Geometry check sheet. Reference: drawing and pictorial views, mm from the part's lowest x, y, z. Coordinates: 2 decimals unless noted, no trailing zeros. Loops run counter-clockwise (first coordinate to the right, second up) from the corner with the lowest first, then second, coordinate; pieces in that order, holes last. Notation, with made-up numbers: (16, 65) -> (44, 65) arc R28 ccw to (44, 102) -> close; hole circle Ø1 at (48, 38). An arc over 180 degrees is marked (long way). Use one line per item in the form item = value.
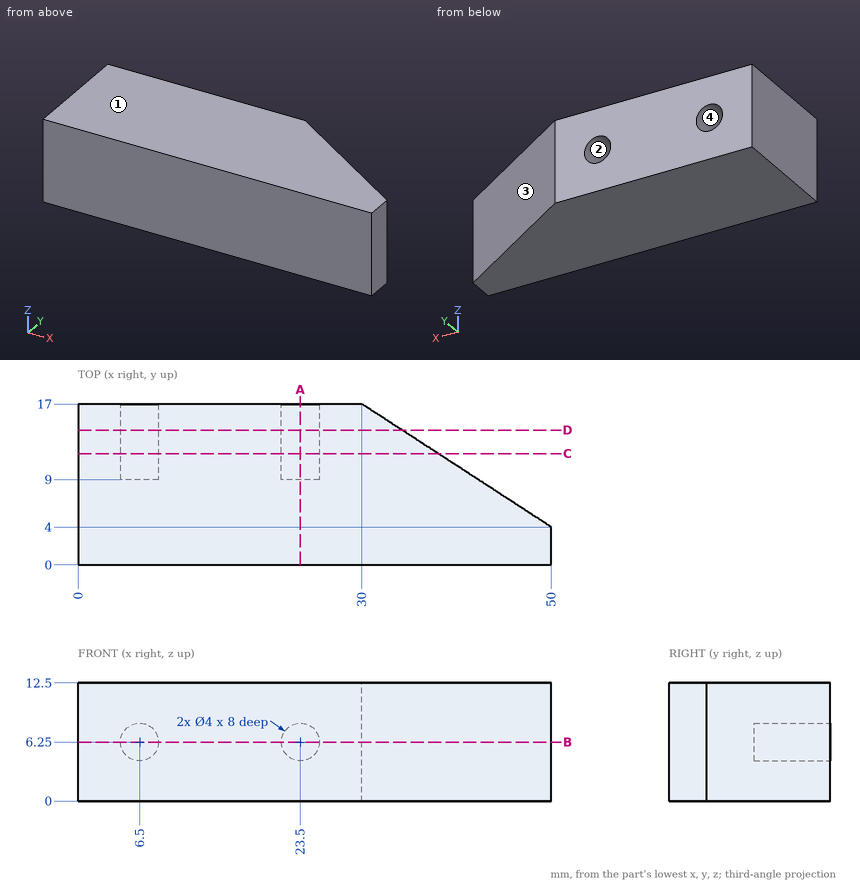
(1) Go/stop test with flat-tipped pins: P1, Ø4, axis at x = 42.5, z = 8.5, coming from the +Y side (3 decimals); P2, Ø5, axis at x = 39, z = 9, coming from the +Y side (3 decimals); P3, Ø3.5, axis at x = 23.5, z = 6.25, coming from the +Y side. Record where each tip stops, or that it passes through.
Established:
P1 = 10.175
P2 = 12.775
P3 = 9
(2) Section check A-A, the plane x = 23.5. Record the boundary of the cut face in (y, z).
Established:
outline = (0, 0) -> (17, 0) -> (17, 4.25) -> (9, 4.25) -> (9, 8.25) -> (17, 8.25) -> (17, 12.5) -> (0, 12.5) -> close
(3) Section check D-D, the plane y = 14.25. Record the boundary of the cut face in (x, z).
Established:
outline = (0, 0) -> (34.23, 0) -> (34.23, 12.5) -> (0, 12.5) -> close; hole circle Ø4 at (6.5, 6.25); hole circle Ø4 at (23.5, 6.25)
(4) Scan lines: line 1 along Z through (x, y) = (6.5, 11); line 2 along X through (y, z) = (14.5, 6.25); line 3 along X through (y, z) = (12, 6.25). Record each from-to range of solid material in increasing order.
Established:
line_1 = 0 to 4.25, 8.25 to 12.5
line_2 = 0 to 4.5, 8.5 to 21.5, 25.5 to 33.85
line_3 = 0 to 4.5, 8.5 to 21.5, 25.5 to 37.69
(5) Section check B-B, the plane z = 6.25. Record the boundary of the cut face in (x, y), plus the area to 3 significant figures.
Established:
outline = (0, 0) -> (50, 0) -> (50, 4) -> (30, 17) -> (25.5, 17) -> (25.5, 9) -> (21.5, 9) -> (21.5, 17) -> (8.5, 17) -> (8.5, 9) -> (4.5, 9) -> (4.5, 17) -> (0, 17) -> close
area = 656 mm²
(6) Mould release check, pull along X, two halves, no side actions. Record for the marked faces 1, 2, 3 and 4: +X half, -X half, draft (parallel to the pull), parting line (faces both ways), or undercut.
Established:
face_1 = draft
face_2 = undercut
face_3 = +X half
face_4 = undercut
(7) Section check C-C, the plane y = 11.75. Record the boundary of the cut face in (x, z).
Established:
outline = (0, 0) -> (38.08, 0) -> (38.08, 12.5) -> (0, 12.5) -> close; hole circle Ø4 at (6.5, 6.25); hole circle Ø4 at (23.5, 6.25)
